Read the model definition and answer for the solid it produces. Units are mm, in the model's axes. Give positions to 0.01 mm unless a question says otherwise; leave off trailing zeros. Write item = value, one per line. Start each with the question number.
from build123d import *
from OCP.BRepFilletAPI import BRepFilletAPI_MakeChamfer

# Parameters (mm, degrees)
BOSS_EXTRUDE1_START = -0.635
SKETCH3_R           = 9.525
SKETCH3_R_2         = 4.7625
BOSS_EXTRUDE1_DEPTH = 1.27
CHAMFER1_SIZE       = 0.127
CHAMFER1_SIZE2      = 0.073323484
FILLET1_R           = 0.381


with BuildPart() as part:
    # Sketch3 → Boss-Extrude1 (new body)
    with BuildSketch(Plane.XY.offset(BOSS_EXTRUDE1_START)):
        Circle(SKETCH3_R)
        Circle(SKETCH3_R_2, mode=Mode.SUBTRACT)
    extrude(amount=BOSS_EXTRUDE1_DEPTH)

    # Chamfer1: one chamfer whose edges measure the first distance from different faces: ONE call of the kernel's chamfer builder (chamfer() names one face for all edges)
    chamfer1_edges_1 = [part.edges().sort_by_distance(p)[0] for p in [
        (-9.525, 0, 0.635),
    ]]
    chamfer1_side_1 = [part.faces().sort_by_distance(p)[0] for p in [
        (-9.525, 0, 0),
    ]]
    chamfer1_edges_2 = [part.edges().sort_by_distance(p)[0] for p in [
        (-4.7625, 0, 0.635),
    ]]
    chamfer1_side_2 = [part.faces().sort_by_distance(p)[0] for p in [
        (-4.7625, 0, 0),
    ]]
    chamfer1 = BRepFilletAPI_MakeChamfer(part.part.solid().wrapped)
    for e in chamfer1_edges_1:
        chamfer1.Add(CHAMFER1_SIZE, CHAMFER1_SIZE2, e.wrapped, chamfer1_side_1[0].wrapped)  # the first distance lies on this face
    for e in chamfer1_edges_2:
        chamfer1.Add(CHAMFER1_SIZE, CHAMFER1_SIZE2, e.wrapped, chamfer1_side_2[0].wrapped)  # the first distance lies on this face
    add(Compound.cast(chamfer1.Shape()), mode=Mode.REPLACE)

    # Fillet1
    # the kernel refuses this fillet: 0.381 mm, written as the material it takes off along each edge
    with BuildSketch(Plane(origin=(0, 0, 0.635), x_dir=(1, 0, 0), z_dir=(0, -1, 0))) as fillet1_piece_1:
        with BuildLine():
            CenterArc((9.241019367, -0.381), FILLET1_R, 41.810314896, 48.189685104)
            Line((9.241019367, 0), (9.241019367, 0.00762))
            Line((9.241019367, 0.00762), (9.451676516, 0.00762))
            Line((9.451676516, 0.00762), (9.458275629, 0.00381))
            ThreePointArc((9.458275629, 0.00381), (9.494937371, -0.05969), (9.530679613, -0.12192))
            Line((9.530679613, -0.12192), (9.525, -0.127))
        make_face()
    revolve(axis=Axis((0, 0, 0.635), (0, 0, 1)), mode=Mode.SUBTRACT)
    with BuildSketch(Plane(origin=(0, 0, 0.635), x_dir=(1, 0, 0), z_dir=(0, -1, 0))) as fillet1_piece_2:
        with BuildLine():
            CenterArc((5.046480633, -0.381), FILLET1_R, 90, 48.189685104)
            Line((4.7625, -0.127), (4.756820387, -0.12192))
            ThreePointArc((4.756820387, -0.12192), (4.792562629, -0.05969), (4.829224371, 0.00381))
            Line((4.829224371, 0.00381), (4.835823484, 0.00762))
            Line((4.835823484, 0.00762), (5.046480633, 0.00762))
            Line((5.046480633, 0.00762), (5.046480633, 0))
        make_face()
    revolve(axis=Axis((0, 0, 0.635), (0, 0, 1)), mode=Mode.SUBTRACT)


solid = part.part
1. Consider line 1 along Y through (x, z) = (0, 0) (1 decimal); line 2 along Y through (x, z) = (2.25, -0.45); line 3 along X through (y, z) = (-4, -0.2). Determine where each line is inside the solid, lowest interval first. Write a range as [from, to].
2. Given P1, Ø3, axis at x = -2.5, y = -1.5, coming from the +Z side, flat-ended and moving along its own axis, determine where the tip first touches the part or whether it passes through.
3. For a pull along X with two mould halves and no side action, classify faces 1 (the flat face through (4, -4, 0.635)), 2 (the cylindrical face through (-7.559, -5.796, -0.072)), 3 (the cylindrical face through (-3.78, -2.9, -0.07)) as released by +X, released by -X, zero draft, split by the parting line, or undercut.
Reply:
q1.line_1 = [-9.5, -4.8], [4.8, 9.5]
q1.line_2 = [-9.26, -4.2], [4.2, 9.26]
q1.line_3 = [-8.64, -2.58], [2.58, 8.64]
q2.P1 = through
q3.face_1 = zero draft
q3.face_2 = split by the parting line
q3.face_3 = undercut
